Check sheet for the modelled part. Datum: model origin and axes. Units: mm. Face numbers are marked on the shaded views. A direction names the side the tool comes from. Give positions to 0.01 mm unless a question says otherwise; leave off trailing zeros. Order: outer loops, then holes, each group sorted by start corner. A loop starts at its lowest first (then second) coordinate and runs counter-clockwise, first axis right, second up.
```python
from build123d import *

# Parameters (mm, degrees)
FILLET1_R           = 1.524
BOSS_EXTRUDE1_START = -13.716
BOSS_EXTRUDE1_DEPTH = 13.716


with BuildPart() as part:
    # Sketch1 → Base-Revolve (revolve)
    with BuildSketch(Plane.XY, mode=Mode.PRIVATE) as base_revolve_sk:
        Polygon((10.414, 39.386322837), (9.6266, 39.386322837), (9.6266, 40.910322837), (7.9502, 40.910322837), (7.9502, 27.194322837), (6.096, 27.194322837), (6.096, 42.434322837), (12.9032, 42.434322837), (12.9032, 40.910322837), (10.414, 40.910322837), align=None)
    revolve(base_revolve_sk.sketch.rotate(Axis((0, 42.434322837, 0), (0, -1, 0)), 90), axis=Axis((0, 42.434322837, 0), (0, -1, 0)))

    # Fillet1
    fillet1_edges = [part.edges().sort_by_distance(p)[0] for p in [
        (0, 42.434322837, -12.9032),
    ]]
    fillet(fillet1_edges, radius=FILLET1_R - 0.0001)  # a hair under: the kernel refuses the full size

    # Sketch3 → Boss-Extrude1 (add)
    with BuildSketch(Plane.XZ.offset(-27.194322837).offset(BOSS_EXTRUDE1_START)):
        with BuildLine():
            Line((-1.166541413, 7.864150378), (-1.166541413, 8.8138))
            Line((-1.166541413, 8.8138), (1.166541413, 8.8138))
            Line((1.166541413, 8.8138), (1.166541413, 7.864150378))
            ThreePointArc((1.166541413, 7.864150378), (0, 7.9502), (-1.166541413, 7.864150378))
        make_face()
    extrude(amount=BOSS_EXTRUDE1_DEPTH)


solid = part.part
```
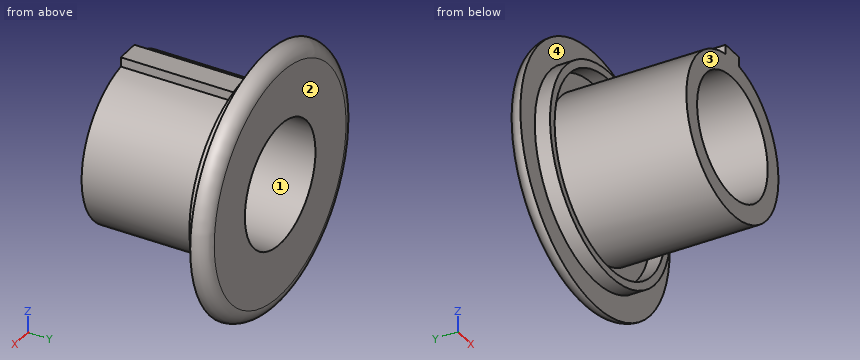
Q1. Go/stop test with flat-tipped pins: P1, Ø0.5, axis at y = 36.5, z = 8.5, coming from the -X side; P2, Ø4, axis at y = 30, z = -5, coming from the -X side; P3, Ø10, axis at x = 0, z = 0, coming from the -Y side; P4, Ø4, axis at x = 4.5, y = 31.5, coming from the -Z side. Record where each tip stops, or that it passes through.
Q2. Material ranges on line 1 (X direction, y = 37.5, z = 0); line 2 (Z direction, x = 1.25, y = 40.5); line 3 (Y direction, x = 6, z = 6.5), recorded low to high.
Q3. Tool access check on the marked faces 3 and 4. Record the directions out of +Z, -Z, +X, -X, +Y, -Y that give a thin tool (end or side, any length) a straight path to the whole face; none if there is none.
Q4. Sectioned sample at C-C, the plane y = 32.5. Record the cut outline in (x, z), plus the area to 3 significant figures.
Q5. Draft check along Z on the marked faces 1 and 2. Enter one of: pulls with the +Z half, pulls with the -Z half, needs draft (parallel to the pull), parting line crosses it, or undercut.
Filled in:
1. P1: stops at x = -1.17
1. P2: stops at x = -7.36
1. P3: passes through
1. P4: stops at z = -7.55
2. line 1: x = -7.95 to -6.1, 6.1 to 7.95
2. line 2: z = -10.34 to -9.55, -7.85 to -5.97, 5.97 to 7.85, 9.55 to 10.34
2. line 3: y = 40.91 to 42.43
3. face 3: +Z, -Z, +X, -X, -Y
3. face 4: -Y
4. outline: (-1.17, 7.86) arc R7.95 ccw (long way) to (1.17, 7.86) - (1.17, 8.81) - (-1.17, 8.81) - close; hole circle Ø12.19 at (0, 0)
4. area: 83.9 mm2
5. face 1: undercut
5. face 2: needs draft
